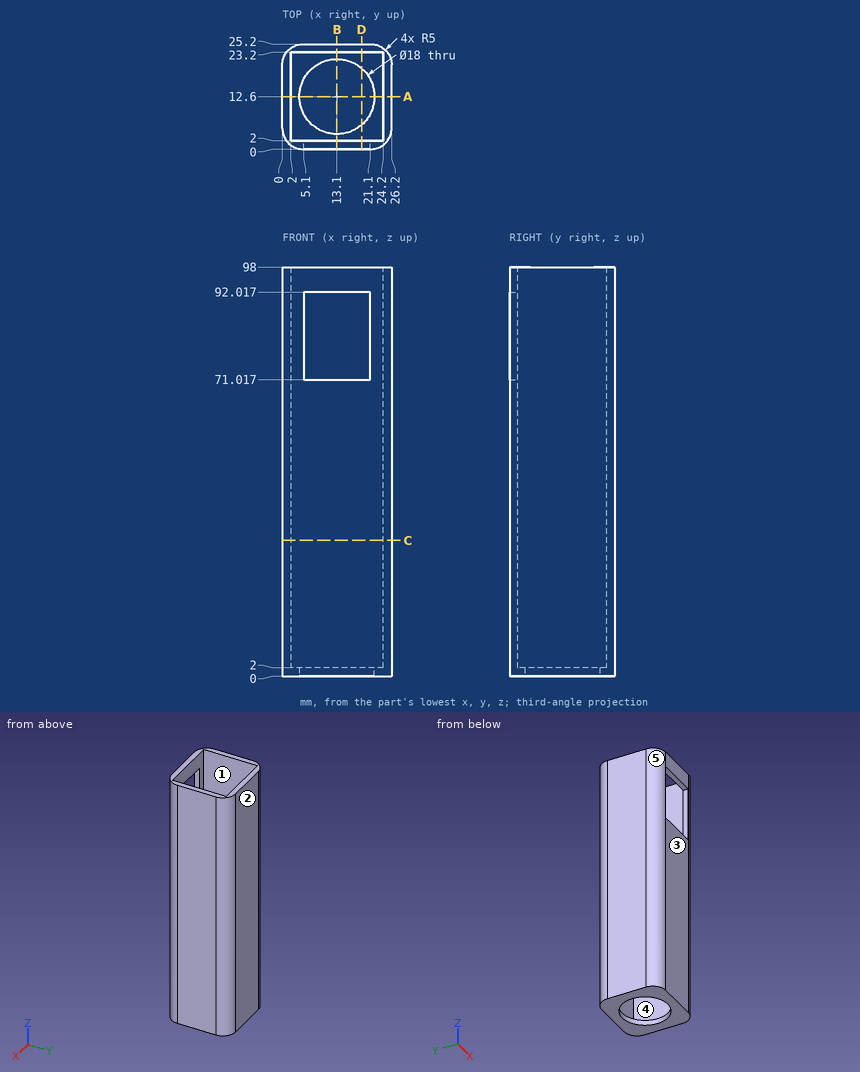
Here's the drawing with two shaded views (mm, measured from the low corner). I have some questions. A direction names the side the tool comes from. Coordinates: 2 decimals unless noted, no trailing zeros. Write each loop counter-clockwise with the first axis right and the second up, starting at its lowest first coordinate (ties: lowest second). Pieces come first, ordered by that corner, then holes. Notation, with made-up numbers: (2, 51) -> (23, 51) arc R18 cw to (23, 60) -> close; hole circle Ø9 at (80.25, -36). An arc over 180 degrees is marked (long way). Write item = value, one per line. Start each with the question number.
(1) I need wall thicknesses on line 1 (X direction, y = 8, z = 15.5); line 2 (Y direction, x = 13.1, z = 1.4); line 3 (Y direction, x = 15.25, z = 19). Which ranges of each line are inside material? Lowest first, please. Write a range as [from, to].
(2) Will these pins go through, and if not, where does the flat tip stop? pin 1 (10.5 mm diameter, centred on x = 18, y = 7.5, fed in from +Z); pin 2 (0.6 mm diameter, centred on y = 1.5, z = 85, fed in from -X); pin 3 (1.6 mm diameter, centred on y = 1, z = 80, fed in from +X).
(3) I want a section at A-A (y = 12.6). Please give me the cut outline in (x, z).
(4) We'd pull the mould along Y, two halves only. Please class the marked faces 1, 2 and 3: released by +Y, released by -Y, zero draft, split by the parting line, or undercut.
(5) I want a section at B-B (x = 13.1). Please give me the cut outline in (y, z).
(6) Which directions (+Z, -Z, +X, -X, +Y, -Y) give clear straight access to the entire face, cutting with the end or side of a thin tool? Please do the marked faces 4 and 5.
(7) I want a section at D-D (x = 19). Please give me the cut outline in (y, z), plus the area to 3 significant figures.
(8) I want a section at C-C (z = 32.5). Please give me the cut outline in (x, y), plus the area to 3 significant figures.
Result set:
q1.line_1 = [0, 2], [24.2, 26.2]
q1.line_2 = [0, 3.6], [21.6, 25.2]
q1.line_3 = [0, 2], [23.2, 25.2]
q2.pin_1 = 2
q2.pin_2 = 1.16
q2.pin_3 = 25.04
q3.outline = (0, 0) -> (4.1, 0) -> (4.1, 2) -> (2, 2) -> (2, 98) -> (0, 98) -> close; (22.1, 0) -> (26.2, 0) -> (26.2, 98) -> (24.2, 98) -> (24.2, 2) -> (22.1, 2) -> close
q4.face_1 = undercut
q4.face_2 = released by +Y
q4.face_3 = released by -Y
q5.outline = (0, 0) -> (3.6, 0) -> (3.6, 2) -> (2, 2) -> (2, 71.02) -> (0, 71.02) -> close; (0, 92.02) -> (2, 92.02) -> (2, 98) -> (0, 98) -> close; (21.6, 0) -> (25.2, 0) -> (25.2, 98) -> (23.2, 98) -> (23.2, 2) -> (21.6, 2) -> close
q6.face_4 = +Z
q6.face_5 = +Z, -Z, -X, -Y
q7.outline = (0, 0) -> (5.8, 0) -> (5.8, 2) -> (2, 2) -> (2, 71.02) -> (0, 71.02) -> close; (0, 92.02) -> (2, 92.02) -> (2, 98) -> (0, 98) -> close; (19.4, 0) -> (25.2, 0) -> (25.2, 98) -> (23.2, 98) -> (23.2, 2) -> (19.4, 2) -> close
q7.area = 365 mm2
q8.outline = (0, 5) arc R5 ccw to (5, 0) -> (21.2, 0) arc R5 ccw to (26.2, 5) -> (26.2, 20.2) arc R5 ccw to (21.2, 25.2) -> (5, 25.2) arc R5 ccw to (0, 20.2) -> close; hole (2, 2) -> (24.2, 2) -> (24.2, 23.2) -> (2, 23.2) -> close
q8.area = 168 mm2
